For this review, use the dimensioned drawing (mm, ordinates from the lowest corner) and the shaded views. A direction names the side the tool comes from. Give positions to 0.01 mm unless a question says otherwise; leave off trailing zeros. Write each loop counter-clockwise with the first axis right and the second up, starting at its lowest first coordinate (ties: lowest second). Pieces come first, ordered by that corner, then holes. Notation, with made-up numbers: M 5.5,-23 L 54.5,-23 A15 cw 54.5,1 Z; hole C -14.5,71.25 d6. An arc over 180 degrees is marked long. One line per item, written item: value. Start each with the question number.
Item 1: Tool access review of the marked faces 4, 5, 6, 7 and 8: name each direction out of +Z, -Z, +X, -X, +Y, -Y from which nothing blocks a thin tool from reaching the whole face with its end or side.
Item 2: To check wall thickness, follow probe 1 along Z at (x, y) = (1.75, 29); probe 2 along Y at (x, z) = (8, 24.5); probe 3 along Z at (x, y) = (2, 8). State the ranges of each line that lie inside material, in increasing order.
Item 3: Consider section A-A, the plane y = 21. Write out the cut boundary in (x, z) (1 decimal).
Item 4: Clearance check with flat-ended pins moving along their axes: pin 1 Ø4 at (x, z) = (2.5, 10.5) entering from +Y; pin 2 Ø1.4 at (x, z) = (1, 12.5) entering from +Y; pin 3 Ø5 at (x, z) = (9, 6.5) entering from -Y. State where each tip first meets the part, or that it passes through.
Item 5: Mouldability with a two-part tool opening along Z and no side actions: class the marked faces 1, 2 and 3 as released by +Z, released by -Z, zero draft, split by the parting line, or undercut.
Item 6: Consider section D-D, the plane z = 20.25. Write out the cut boundary in (x, y).
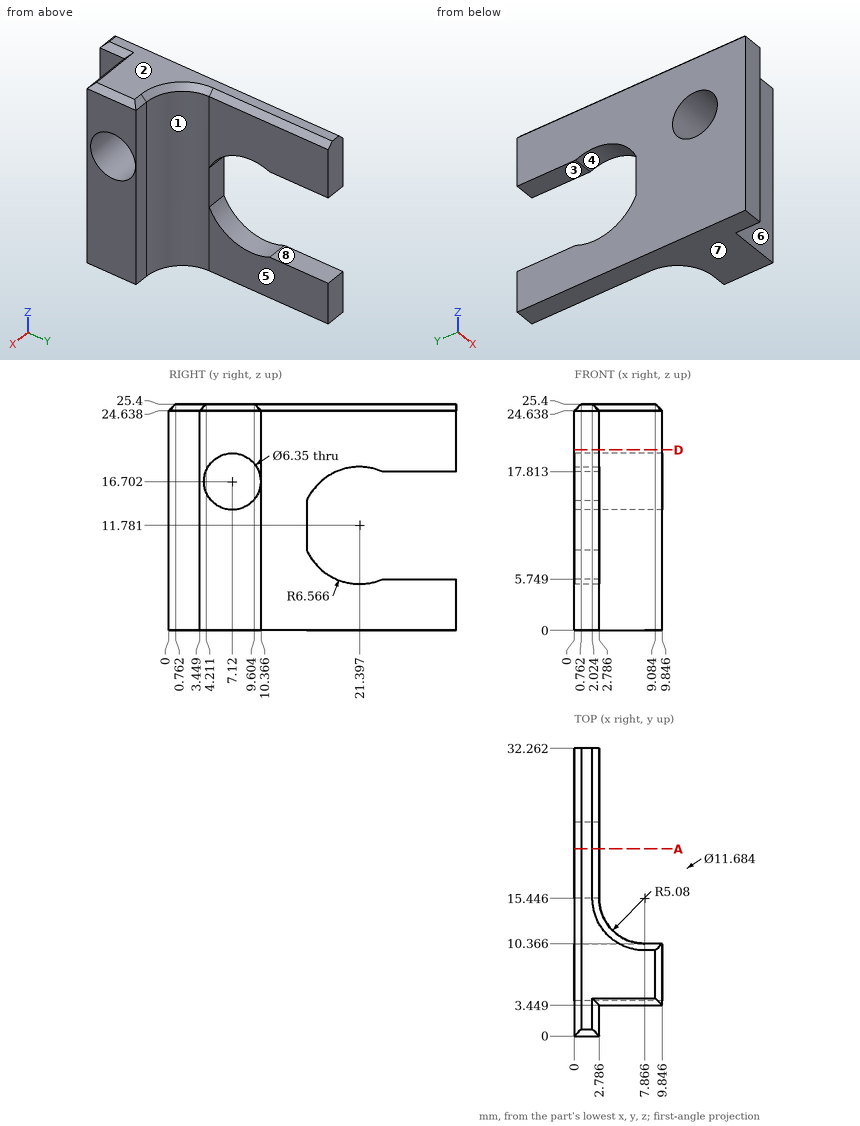
Model answer:
1. face 4: +X, -X
1. face 5: +Z, -Z, +X, +Y
1. face 6: +Z, -Z, +X, -Y
1. face 7: -Z, +X, -X, +Y, -Y
1. face 8: +X, -X, +Y
2. probe 1: z = 0 to 5.75, 17.81 to 25.4
2. probe 2: y = 3.45 to 10.37
2. probe 3: z = 0 to 13.65, 19.75 to 25.4
3. outline: M 0,0 L 2.8,0 L 2.8,5.2 L 0,5.2 Z; M 0,18.3 L 2.8,18.3 L 2.8,24.6 L 2,25.4 L 0.8,25.4 L 0,24.6 Z
4. pin 1: stops at y = 15.71
4. pin 2: stops at y = 15.45
4. pin 3: stops at y = 3.45
5. face 1: zero draft
5. face 2: released by +Z
5. face 3: undercut
6. outline: M 0,0 L 2.79,0 L 2.79,3.45 L 9.85,3.45 L 9.85,10.37 L 7.87,10.37 A5.08 cw 2.79,15.45 L 2.79,32.26 L 0,32.26 Z
